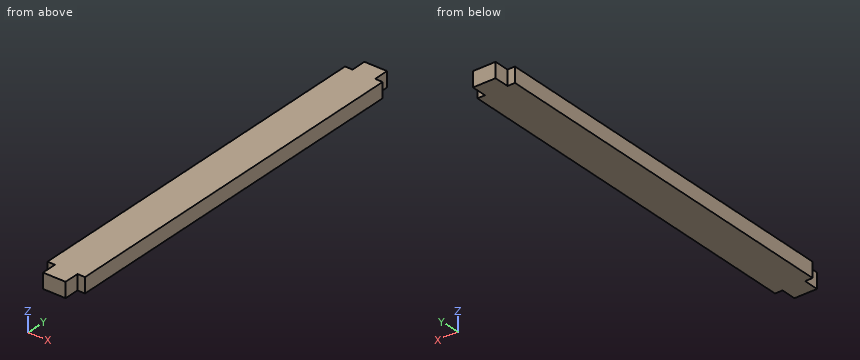
Autodesk Inventor part; units mm, degrees
ref_plane "YZ Plane" through (0, 0, 0) normal (1, 0, 0) x (0, 1, 0)
ref_plane "XZ Plane" through (0, 0, 0) normal (0, 1, 0) x (-1, 0, 0)
ref_plane "XY Plane" through (0, 0, 0) normal (0, 0, 1) x (1, 0, 0)
sketch "Sketch1" plane through (0, 0, 0) normal (0, 0, 1) x (1, 0, 0)
  line L0 (3, 54) -> (-3, 54)
  line L1 (-3, 54) -> (-3, 50)
  line L2 (-3, -54) -> (3, -54)
  line L3 (3, -54) -> (3, -50)
  line L4 (-3, 50) -> (-5, 50)
  line L5 (-5, 50) -> (-5, -50)
  line L6 (-5, -50) -> (-3, -50)
  line L7 (-3, -50) -> (-3, 50) construction
  line L8 (-3, 50) -> (-3, -50) construction
  line L9 (-3, -50) -> (-3, -54)
  line L10 (0, 54) -> (0, -54)
  line L11 (3, 50) -> (5, 50)
  line L12 (5, 50) -> (5, -50)
  line L13 (5, -50) -> (3, -50)
  line L14 (3, 50) -> (3, 54)
  line L15 (3, -50) -> (3, 50) construction
  point P0 (0, 0)
  point P1 (-4, -50)
  point P2 (0, 0)
  point P3 (0, 0)
  dimension "d0" = 6
  dimension "d1" = 108
  dimension "d2" = 4
  dimension "d3" = 4
  dimension "d4" = 2
extrude "Extrusion1" add sketch "Sketch1" along normal blind 4
properties part number "MagnetHolder" material "Wood (Oak)"
Part model, mm, in its own coordinate system. Round coordinates to 2 decimals unless told otherwise and drop trailing zeros. Loops run counter-clockwise (first coordinate to the right, second up) from the corner with the lowest first, then second, coordinate; pieces in that order, holes last. Notation, with made-up numbers: (-16, 54) -> (29, 54) arc R23 ccw to (29, 86) -> close; hole circle Ø6 at (-13.5, -30). An arc over 180 degrees is marked (long way). Use CSV: the item, a comma, the result in double quotes. Start each with the question number.
1) Drop flat-ended pins along their axis: P1, Ø1.2, axis at y = -52, z = 1.5, coming from the +X side; P2, Ø1, axis at x = 4.5, z = 1, coming from the -Y side; P3, Ø1, axis at x = 4.5, z = 2.5, coming from the +Y side. Give the stop position or say it passes through.
2) Wall check: L1, parallel to Y at x = 4.25, z = 1. Give the ranges that are in metal, low to high. Write a range as [from, to].
3) Cut at A-A, the plane z = 3.05. Write the cut outline in (x, y).
Determined:
1,P1,"stops at x = 3"
1,P2,"stops at y = -50"
1,P3,"stops at y = 50"
2,L1,"y = [-50, 50]"
3,outline,"(-5, -50) -> (-3, -50) -> (-3, -54) -> (3, -54) -> (3, -50) -> (5, -50) -> (5, 50) -> (3, 50) -> (3, 54) -> (-3, 54) -> (-3, 50) -> (-5, 50) -> close"
